The figure shows three views and two pictorial views of one solid part (mm, origin at its lowest corner). Answer the questions. Give positions to 0.01 mm unless a question says otherwise; leave off trailing zeros. Loops run counter-clockwise (first coordinate to the right, second up) from the corner with the lowest first, then second, coordinate; pieces in that order, holes last. Notation, with made-up numbers: (58, 71) - (64, 71) arc R36 ccw to (64, 107) - close; hole circle Ø8 at (48, -34). An arc over 180 degrees is marked (long way). Use a Markdown table: item, result. Add a question column.
Item 1: Consider probe 1 along Y at (x, z) = (201, 4.5) (3 decimals); probe 2 along Z at (x, y) = (277.5, 21.75) (3 decimals); probe 3 along Y at (x, z) = (311, 2). Determine where each line is inside the solid, lowest interval first. Write a range as [from, to].
Item 2: A cutting plane is placed at A-A (z = 43). Determine the outline of the cut face in (x, y) (3 decimals), plus the area to 3 significant figures.
Item 3: A cutting plane is placed at D-D (x = 277.5). Determine the outline of the cut face in (y, z) (3 decimals).
Item 4: A cutting plane is placed at B-B (y = 19). Determine the outline of the cut face in (x, z) (3 decimals), plus the area to 3 significant figures.
Item 5: A cutting plane is placed at C-C (x = 88.9). Determine the outline of the cut face in (y, z) (3 decimals), plus the area to 3 significant figures.
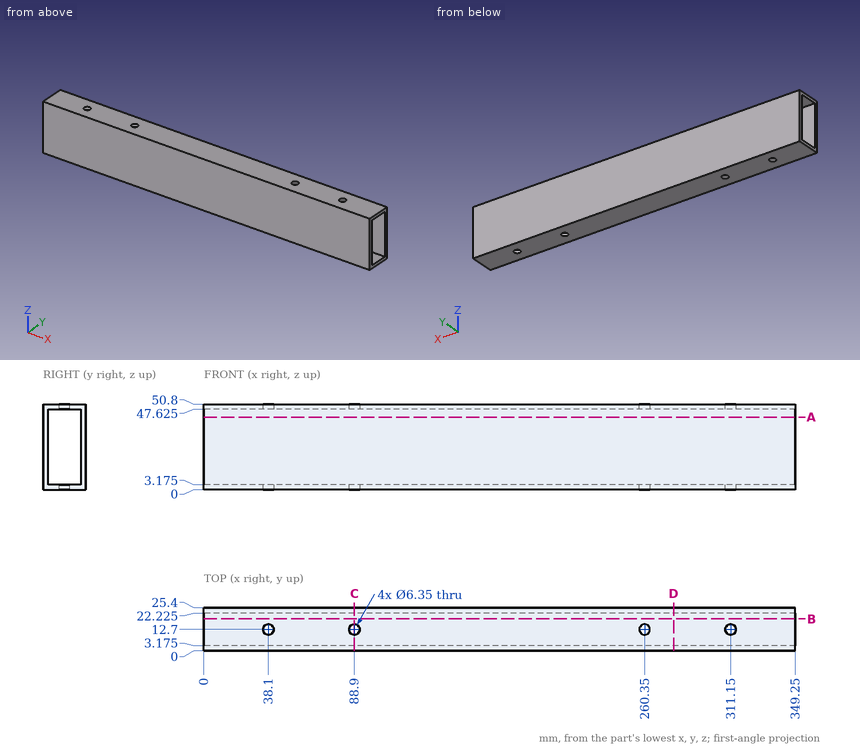
Geometry says:
| question | item | result |
|---|---|---|
| 1 | probe 1 | [0, 3.175], [22.225, 25.4] |
| 1 | probe 2 | [0, 3.175], [47.625, 50.8] |
| 1 | probe 3 | [0, 9.53], [15.87, 25.4] |
| 2 | outline | (0, 0) - (349.25, 0) - (349.25, 3.175) - (0, 3.175) - close; (0, 22.225) - (349.25, 22.225) - (349.25, 25.4) - (0, 25.4) - close |
| 2 | area | 2,220 mm² |
| 3 | outline | (0, 0) - (25.4, 0) - (25.4, 50.8) - (0, 50.8) - close; hole (3.175, 3.175) - (22.225, 3.175) - (22.225, 47.625) - (3.175, 47.625) - close |
| 4 | outline | (0, 0) - (349.25, 0) - (349.25, 3.175) - (0, 3.175) - close; (0, 47.625) - (349.25, 47.625) - (349.25, 50.8) - (0, 50.8) - close |
| 4 | area | 2,220 mm² |
| 5 | outline | (0, 0) - (9.525, 0) - (9.525, 3.175) - (3.175, 3.175) - (3.175, 47.625) - (9.525, 47.625) - (9.525, 50.8) - (0, 50.8) - close; (15.875, 0) - (25.4, 0) - (25.4, 50.8) - (15.875, 50.8) - (15.875, 47.625) - (22.225, 47.625) - (22.225, 3.175) - (15.875, 3.175) - close |
| 5 | area | 403 mm² |
